```python
from build123d import *

# Parameters (mm, degrees)
SKETCH1_W          = 3
SKETCH1_H          = 45
REVOLVE1_ANGLE     = 180
SKETCH2_R          = 1.5
CUT_EXTRUDE1_DEPTH = 10


with BuildPart() as part:
    # Sketch1 → Revolve1 (revolve)
    with BuildSketch(Plane(origin=(0, 0, 0), x_dir=(1, 0, 0), z_dir=(0, 1, 0))):
        Rectangle(SKETCH1_W, SKETCH1_H)
    revolve(axis=Axis((-51.5, 0, -27.834324949), (0, 0, 1)), revolution_arc=REVOLVE1_ANGLE)

    # Sketch2 → Cut-Extrude1 (cut)
    with BuildSketch(Plane(origin=(0, 54, 0), x_dir=(1, 0, 0), z_dir=(0, 1, 0))):
        with Locations(Location((-52.203545166, 0, 0), (0, 0, 270))):
            Circle(SKETCH2_R)
    extrude(amount=-CUT_EXTRUDE1_DEPTH, mode=Mode.SUBTRACT)


solid = part.part
```
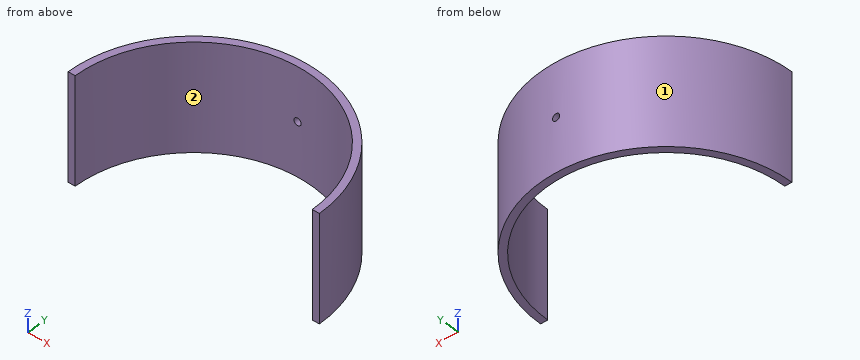
Work out the finished part from the listing and answer in its coordinate system (mm). Face numbers are marked on the shaded views. Give positions to 0.01 mm unless a question says otherwise; leave off trailing zeros. Write each loop counter-clockwise with the first axis right and the second up, starting at its lowest first coordinate (ties: lowest second). Pieces come first, ordered by that corner, then holes. Notation, with made-up numbers: (66.5, 73.5) -> (71.5, 73.5) arc R20 ccw to (71.5, 111.5) -> close; hole circle Ø2 at (5, 36.25). An arc over 180 degrees is marked (long way). Write item = value, one per line.
Q1. For a pull along X with two mould halves and no side action, classify the marked faces 1 and 2 as pulls with the +X half, pulls with the -X half, needs draft (parallel to the pull), parting line crosses it, or undercut.
Computed values:
face_1 = parting line crosses it
face_2 = undercut
Q2. Section C-C on y = 42 is taken. Determine the outline of the cut face in (x, z), and give its area (3 significant figures).
Computed values:
outline = (-83.83, -22.5) -> (-78.63, -22.5) -> (-78.63, 22.5) -> (-83.83, 22.5) -> close; (-24.37, -22.5) -> (-19.17, -22.5) -> (-19.17, 22.5) -> (-24.37, 22.5) -> close
area = 468 mm^2
Q3. Section D-D on x = -9 is taken. Determine the outline of the cut face in (y, z).
Computed values:
outline = (26.34, -22.5) -> (31.67, -22.5) -> (31.67, 22.5) -> (26.34, 22.5) -> close
Q4. Consider line 1 along X through (y, z) = (24, -3); line 2 along X through (y, z) = (29, 5.5); line 3 along Y through (x, z) = (-88, 16.5). Determine where each line is inside the solid, lowest interval first.
Computed values:
line_1 = -98.75 to -95.36, -7.64 to -4.25
line_2 = -95.86 to -92.23, -10.77 to -7.14
line_3 = 34.17 to 38.43
Q5. Flat-ended cylindrical pins translate along their axes: pin 1 Ø3 at (y, z) = (39.5, 11) entering from -X; pin 2 Ø1 at (x, z) = (-35.5, -14.5) entering from +Y; pin 3 Ø3.5 at (x, z) = (-52.2, 0) entering from -Y. Find the tip coordinate at first contact, or state that the pin passes through.
Computed values:
pin_1 = -88.45
pin_2 = 50.68
pin_3 = 49.94
Q6. Section B-B on z = -9 is taken. Determine the outline of the cut face in (x, y), and give its area (3 significant figures).
Computed values:
outline = (-104.5, 0) -> (-101.5, 0) arc R50 cw to (-1.5, 0) -> (1.5, 0) arc R53 ccw to start
area = 485 mm^2
Q7. Section A-A on y = 33 is taken. Determine the outline of the cut face in (x, z).
Computed values:
outline = (-92.97, -22.5) -> (-89.06, -22.5) -> (-89.06, 22.5) -> (-92.97, 22.5) -> close; (-13.94, -22.5) -> (-10.03, -22.5) -> (-10.03, 22.5) -> (-13.94, 22.5) -> close
